```python
from build123d import *

# Parameters (mm, degrees)
SKETCH1_W                = 85
SKETCH1_H                = 45
BOSS_EXTRUDE1_DEPTH      = 5
CUT_EXTRUDE1_OUTLINE_R   = 2
CUT_EXTRUDE1_OUTLINE_R_2 = 2.5
CUT_EXTRUDE1_DEPTH       = 5
SKETCH3_W                = 85
SKETCH3_H                = 45
CUT_EXTRUDE2_DEPTH       = 1


# Read off the part's stored shape, not the designer's step: Cut-Extrude1
with BuildPart() as part:
    # Sketch1 → Boss-Extrude1 (new body)
    with BuildSketch(Plane.XY):
        with Locations((-42.5, 22.5)):
            Rectangle(SKETCH1_W, SKETCH1_H)
    extrude(amount=BOSS_EXTRUDE1_DEPTH)

    # Cut-Extrude1 outline → Cut-Extrude1 (cut)
    with BuildSketch(Plane.XY):
        with Locations((-81, 40)):
            Circle(CUT_EXTRUDE1_OUTLINE_R)
        with Locations((-35, 5)):
            Circle(CUT_EXTRUDE1_OUTLINE_R)
        with Locations((-35, 40)):
            Circle(CUT_EXTRUDE1_OUTLINE_R)
        with Locations((-4, 40)):
            Circle(CUT_EXTRUDE1_OUTLINE_R)
        with Locations((-42.5, 22.5)):
            Circle(CUT_EXTRUDE1_OUTLINE_R_2)
        with Locations((-81, 5)):
            Circle(CUT_EXTRUDE1_OUTLINE_R)
        with Locations((-50, 5)):
            Circle(CUT_EXTRUDE1_OUTLINE_R)
        with Locations((-50, 40)):
            Circle(CUT_EXTRUDE1_OUTLINE_R)
        with Locations((-4, 5)):
            Circle(CUT_EXTRUDE1_OUTLINE_R)
    extrude(amount=CUT_EXTRUDE1_DEPTH, mode=Mode.SUBTRACT)

    # Sketch3 → Cut-Extrude2 (cut)
    with BuildSketch(Plane.XY.offset(5)):
        with Locations((-42.5, 22.5)):
            Rectangle(SKETCH3_W, SKETCH3_H)
    extrude(amount=-CUT_EXTRUDE2_DEPTH, mode=Mode.SUBTRACT)


solid = part.part
```
For this review, take the finished solid that the model builds, in its own axes (mm). Round coordinates to 2 decimals unless told otherwise and drop trailing zeros. Write each loop counter-clockwise with the first axis right and the second up, starting at its lowest first coordinate (ties: lowest second). Pieces come first, ordered by that corner, then holes. Notation, with made-up numbers: (0.25, 68.25) - (41.25, 68.25) arc R7 ccw to (41.25, 76.25) - close; hole circle Ø6 at (-36, 23.5). An arc over 180 degrees is marked (long way). Answer as CSV lines item,"result". Start each with the question number.
(1) Add section B-B, the plane y = 5. State the section outline as (x, z) points.
(2) Add section D-D, the plane z = 1.7. State how many separate pieces and enclosed holes the cut face has, plus the area to 3 significant figures.
(3) Add section C-C, the plane y = 22.5. State the section outline as (x, z) points.
(4) For line 1 (Y direction, x = -50, z = 2.5); line 2 (X direction, y = 5, z = 2.8); line 3 (X direction, y = 39.5, z = 0.2), list the stretches that pass through material, from the lowest coordinate up.
(5) Add section A-A, the plane x = -50. State the section outline as (y, z) points.
(6) Mouldability with a two-part tool opening along Y and no side actions: class faces 1 (the flat face through (-43, 0, 2)), 2 (the cylindrical face through (-52, 5, 2)), 3 (the flat face through (0, 22, 2)) as +Y half, -Y half, draft (parallel to the pull), parting line (faces both ways), or undercut.
(7) For pin 1 (5 mm diameter, centred on x = -50, y = 5, fed in from +Z), flat-tipped, find the tip position at first contact; note if it passes through.
From the geometry:
1,outline,"(-85, 0) - (-83, 0) - (-83, 4) - (-85, 4) - close; (-79, 0) - (-52, 0) - (-52, 4) - (-79, 4) - close; (-48, 0) - (-37, 0) - (-37, 4) - (-48, 4) - close; (-33, 0) - (-6, 0) - (-6, 4) - (-33, 4) - close; (-2, 0) - (0, 0) - (0, 4) - (-2, 4) - close"
2,separate pieces,"1"
2,enclosed holes,"9"
2,area,"3,700 mm²"
3,outline,"(-85, 0) - (-45, 0) - (-45, 4) - (-85, 4) - close; (-40, 0) - (0, 0) - (0, 4) - (-40, 4) - close"
4,line 1,"y = 0 to 3, 7 to 38, 42 to 45"
4,line 2,"x = -85 to -83, -79 to -52, -48 to -37, -33 to -6, -2 to 0"
4,line 3,"x = -85 to -82.94, -79.06 to -51.94, -48.06 to -36.94, -33.06 to -5.94, -2.06 to 0"
5,outline,"(0, 0) - (3, 0) - (3, 4) - (0, 4) - close; (7, 0) - (38, 0) - (38, 4) - (7, 4) - close; (42, 0) - (45, 0) - (45, 4) - (42, 4) - close"
6,face 1,"-Y half"
6,face 2,"undercut"
6,face 3,"draft"
7,pin 1,"stops at z = 4"
